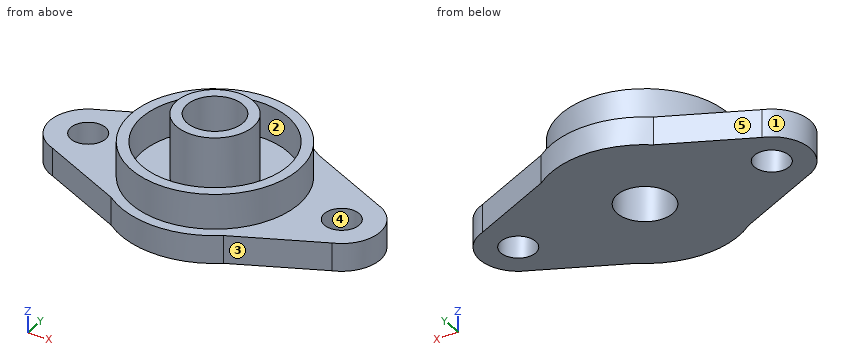
from build123d import *

# Parameters (mm, degrees)
ESBO_O1_R                = 4
ESBO_O1_R_2              = 2.5
RESSALTO_EXTRUS_O1_DEPTH = 4
ESBO_O2_R                = 12.015701032
ESBO_O2_R_2              = 10.48384183
RESSALTO_EXTRUS_O2_DEPTH = 5
ESBO_O3_R                = 5.5
ESBO_O3_R_2              = 4
RESSALTO_EXTRUS_O3_DEPTH = 9


with BuildPart() as part:
    # Esboço1 → Ressalto-extrusão1 (new body)
    with BuildSketch(Plane.XY):
        with BuildLine():
            Line((-20.12399727, 5.170892982), (-8.093718556, 10.80470823))
            ThreePointArc((-8.093718556, 10.80470823), (0, 13.5), (8.093718556, 10.80470823))
            Line((8.093718556, 10.80470823), (20.12399727, 5.170892982))
            ThreePointArc((20.12399727, 5.170892982), (23.75, 0), (20.12399727, -5.170892982))
            Line((20.12399727, -5.170892982), (8.093718556, -10.80470823))
            ThreePointArc((8.093718556, -10.80470823), (0, -13.5), (-8.093718556, -10.80470823))
            Line((-8.093718556, -10.80470823), (-20.12399727, -5.170892982))
            ThreePointArc((-20.12399727, -5.170892982), (-23.75, 0), (-20.12399727, 5.170892982))
        make_face()
        Circle(ESBO_O1_R, mode=Mode.SUBTRACT)
        with Locations((-18.25, 0)):
            Circle(ESBO_O1_R_2, mode=Mode.SUBTRACT)
        with Locations((18.25, 0)):
            Circle(ESBO_O1_R_2, mode=Mode.SUBTRACT)
    extrude(amount=RESSALTO_EXTRUS_O1_DEPTH)

    # Esboço2 → Ressalto-extrusão2 (add)
    with BuildSketch(Plane.XY.offset(4)):
        Circle(ESBO_O2_R)
        Circle(ESBO_O2_R_2, mode=Mode.SUBTRACT)
    extrude(amount=RESSALTO_EXTRUS_O2_DEPTH)

    # Esboço3 → Ressalto-extrusão3 (add)
    with BuildSketch(Plane.XY.offset(4)):
        Circle(ESBO_O3_R)
        Circle(ESBO_O3_R_2, mode=Mode.SUBTRACT)
    extrude(amount=RESSALTO_EXTRUS_O3_DEPTH)


solid = part.part
Can you work these out from the model? Positions are in its coordinate system, mm. Face numbers are marked on the shaded views. A direction names the side the tool comes from. Give positions to 0.01 mm unless a question says otherwise; leave off trailing zeros. Loops run counter-clockwise (first coordinate to the right, second up) from the corner with the lowest first, then second, coordinate; pieces in that order, holes last. Notation, with made-up numbers: (71, 9) - (77, 9) arc R21 cw to (77, 33) - close; hole circle Ø8 at (-12.75, 0). An arc over 180 degrees is marked (long way). Answer as a JSON object with one key per item and string values.
Q1. Which directions (+Z, -Z, +X, -X, +Y, -Y) give clear straight access to the entire face, cutting with the end or side of a thin tool? Please do the marked faces 1 and 2.
Geometry says:
{"face 1": "+Z, -Z, -X", "face 2": "+Z"}
Q2. If we mould it in two halves opening along X, with no side actions, what happens to the marked faces 3, 4 and 5? For each: pulls with the +X half, pulls with the -X half, needs draft (parallel to the pull), parting line crosses it, or undercut.
Geometry says:
{"face 3": "pulls with the +X half", "face 4": "undercut", "face 5": "pulls with the -X half"}
Q3. Will these pins go through, and if not, where does the flat tip stop? P1, Ø6, axis at y = -7, z = 11.5, coming from the +X side; P2, Ø10, axis at x = 10, y = 5, coming from the +Z side; P3, Ø6.5, axis at x = -18.25, y = 0, coming from the +Z side; P4, Ø4, axis at x = 18.25, y = 0, coming from the -Z side.
Geometry says:
{"P1": "x = 10.76", "P2": "z = 9", "P3": "z = 4", "P4": "through"}
Q4. If I drill on L1, parallel to Y at x = 0, z = 6; L2, parallel to Y at x = -2, z = 5.5; L3, parallel to Z at x = 22, y = -1.5, over which ranges is the centre line in solid material (lowest first)?
Geometry says:
{"L1": "-12.02 to -10.48, -5.5 to -4, 4 to 5.5, 10.48 to 12.02", "L2": "-11.85 to -10.29, -5.12 to -3.46, 3.46 to 5.12, 10.29 to 11.85", "L3": "0 to 4"}
Q5. Imagine slicing it at C-C on z = 2.25. Write out the boundary of the cut face in (x, y).
Geometry says:
{"outline": "(-20.12, -5.17) - (-8.09, -10.8) arc R13.5 ccw to (8.09, -10.8) - (20.12, -5.17) arc R5.5 ccw to (20.12, 5.17) - (8.09, 10.8) arc R13.5 ccw to (-8.09, 10.8) - (-20.12, 5.17) arc R5.5 ccw to start; hole circle Ø5 at (-18.25, 0); hole circle Ø8 at (0, 0); hole circle Ø5 at (18.25, 0)"}
Q6. Imagine slicing it at D-D on z = 11.5. Write out the boundary of the cut face in (x, y), plus the area to 3 significant figures.
Geometry says:
{"outline": "circle Ø11 at (0, 0); hole circle Ø8 at (0, 0)", "area": "44.8 mm²"}
Q7. Imagine slicing it at A-A on y = 0. Write out the boundary of the cut face in (x, z), plus the area to 3 significant figures.
Geometry says:
{"outline": "(-23.75, 0) - (-20.75, 0) - (-20.75, 4) - (-23.75, 4) - close; (-15.75, 0) - (-4, 0) - (-4, 13) - (-5.5, 13) - (-5.5, 4) - (-10.48, 4) - (-10.48, 9) - (-12.02, 9) - (-12.02, 4) - (-15.75, 4) - close; (4, 0) - (15.75, 0) - (15.75, 4) - (12.02, 4) - (12.02, 9) - (10.48, 9) - (10.48, 4) - (5.5, 4) - (5.5, 13) - (4, 13) - close; (20.75, 0) - (23.75, 0) - (23.75, 4) - (20.75, 4) - close", "area": "160 mm²"}
Q8. Imagine slicing it at B-B on x = 0. Write out the boundary of the cut face in (y, z).
Geometry says:
{"outline": "(-13.5, 0) - (-4, 0) - (-4, 13) - (-5.5, 13) - (-5.5, 4) - (-10.48, 4) - (-10.48, 9) - (-12.02, 9) - (-12.02, 4) - (-13.5, 4) - close; (4, 0) - (13.5, 0) - (13.5, 4) - (12.02, 4) - (12.02, 9) - (10.48, 9) - (10.48, 4) - (5.5, 4) - (5.5, 13) - (4, 13) - close"}
